For this review, take the finished solid that the model builds, in its own axes (mm). Face numbers are marked on the shaded views. Coordinates: 2 decimals unless noted, no trailing zeros. Write each loop counter-clockwise with the first axis right and the second up, starting at its lowest first coordinate (ties: lowest second). Pieces come first, ordered by that corner, then holes. Notation, with made-up numbers: M 5,-4 L 14,-4 A34 cw 14,34 Z; hole C 38.25,67.25 d2. An arc over 180 degrees is marked long. Return JSON: item names as keys, results as strings.
```python
from build123d import *

# Parameters (mm, degrees)
SKETCH_W        = 134
SKETCH_H        = 62
PAD_DEPTH       = 5
SKETCH001_W     = 134
SKETCH001_H     = 3
PAD001_DEPTH    = 57
SKETCH002_W     = 7
SKETCH002_H     = 17
PAD002_DEPTH    = 7
POCKET_DEPTH    = 89
FILLET_R        = 3
SKETCH004_W     = 3
SKETCH004_H     = 57
PAD003_DEPTH    = 5
SKETCH005_W     = 3
SKETCH005_H     = 7
PAD004_DEPTH    = 3
SKETCH006_R     = 1.75
POCKET001_DEPTH = 134.001
SKETCH007_R     = 1.75
POCKET002_DEPTH = 5
SKETCH008_R     = 1.75
POCKET003_DEPTH = 5
SKETCH009_W     = 3
SKETCH009_H     = 6
PAD005_DEPTH    = 6
SKETCH010_R     = 1.75
POCKET004_DEPTH = 134.001
FILLET001_R     = 3
FILLET002_R     = 2
FILLET003_R     = 3
FILLET004_R     = 2
FILLET005_R     = 6
FILLET006_R     = 6
FILLET007_R     = 2
FILLET008_R     = 0.5
FILLET009_R     = 2
FILLET010_R     = 0.5
FILLET011_R     = 2
FILLET012_R     = 0.5
FILLET013_R     = 2
FILLET014_R     = 0.5
SKETCH011_R     = 1.75
POCKET005_DEPTH = 5
SKETCH012_R     = 2.1
POCKET006_DEPTH = 5
POCKET007_DEPTH = 5
FILLET015_R     = 1
FILLET016_R     = 1


with BuildPart() as part:
    # Sketch → Pad (new body)
    with BuildSketch(Plane.XY):
        with Locations((67, -31)):
            Rectangle(SKETCH_W, SKETCH_H)
    extrude(amount=PAD_DEPTH)

    # Sketch001 (on Face6 of Pad) → Pad001 (join)
    with BuildSketch(Plane.XY.offset(5)):
        with Locations((67, -1.5)):
            Rectangle(SKETCH001_W, SKETCH001_H)
    extrude(amount=PAD001_DEPTH)

    # Sketch002 (on Face11 of Pad001) → Pad002 (join)
    with BuildSketch(Plane.XZ.offset(3)):
        with Locations((26, 53.5)):
            Rectangle(SKETCH002_W, SKETCH002_H)
        with Locations((108, 53.5)):
            Rectangle(SKETCH002_W, SKETCH002_H)
    extrude(amount=PAD002_DEPTH)

    # Sketch003 (on Face14 of Pad002) → Pocket (cut)
    with BuildSketch(Plane(origin=(22.5, 0, 0), x_dir=(0, -1, 0), z_dir=(-1, 0, 0))):
        Polygon((3, 45), (10, 57), (10, 45), align=None)
    extrude(amount=-POCKET_DEPTH, mode=Mode.SUBTRACT)

    # Fillet
    fillet_edges = [part.edges().sort_by_distance(p)[0] for p in [
        (104.5, -10, 59.5),
        (111.5, -10, 59.5),
        (111.5, -6.5, 51),
        (104.5, -6.5, 51),
        (22.5, -10, 59.5),
        (29.5, -10, 59.5),
        (29.5, -6.5, 51),
        (22.5, -6.5, 51),
    ]]
    fillet(fillet_edges, radius=FILLET_R)

    # Sketch004 (on Face1 of Fillet) → Pad003 (join)
    with BuildSketch(Plane.XZ.offset(3)):
        with Locations((1.5, 33.5)):
            Rectangle(SKETCH004_W, SKETCH004_H)
        with Locations((132.5, 33.5)):
            Rectangle(SKETCH004_W, SKETCH004_H)
    extrude(amount=PAD003_DEPTH)

    # Sketch005 (on Face32 of Pad003) → Pad004 (join)
    with BuildSketch(Plane.XZ.offset(8)):
        with Locations((1.5, 8.5)):
            Rectangle(SKETCH005_W, SKETCH005_H)
        with Locations((1.5, 58.5)):
            Rectangle(SKETCH005_W, SKETCH005_H)
        with Locations((132.5, 8.5)):
            Rectangle(SKETCH005_W, SKETCH005_H)
        with Locations((132.5, 58.5)):
            Rectangle(SKETCH005_W, SKETCH005_H)
    extrude(amount=PAD004_DEPTH)

    # Sketch006 (on Face44 of Pad004) → Pocket001 (cut, through all)
    with BuildSketch(Plane(origin=(0, 0, 0), x_dir=(0, -1, 0), z_dir=(-1, 0, 0))):
        with Locations((7, 8)):
            Circle(SKETCH006_R)
    extrude(amount=-POCKET001_DEPTH, mode=Mode.SUBTRACT)

    # Sketch007 (on Face46 of Pocket001) → Pocket002 (cut)
    with BuildSketch(Plane(origin=(0, 0, 0), x_dir=(0, -1, 0), z_dir=(-1, 0, 0))):
        with Locations((7, 58)):
            Circle(SKETCH007_R)
    extrude(amount=-POCKET002_DEPTH, mode=Mode.SUBTRACT)

    # Sketch008 (on Face45 of Pocket002) → Pocket003 (cut)
    with BuildSketch(Plane.YZ.offset(134)):
        with Locations((-7, 58)):
            Circle(SKETCH008_R)
    extrude(amount=-POCKET003_DEPTH, mode=Mode.SUBTRACT)

    # Sketch009 (on Face10 of Pocket003) → Pad005 (join)
    with BuildSketch(Plane.XY.offset(5)):
        with Locations((1.5, -59)):
            Rectangle(SKETCH009_W, SKETCH009_H)
        with Locations((132.5, -59)):
            Rectangle(SKETCH009_W, SKETCH009_H)
    extrude(amount=PAD005_DEPTH)

    # Sketch010 (on Face60 of Pad005) → Pocket004 (cut, through all)
    with BuildSketch(Plane.YZ.offset(134)):
        with Locations((-59, 8)):
            Circle(SKETCH010_R)
    extrude(amount=-POCKET004_DEPTH, mode=Mode.SUBTRACT)

    # Fillet001
    fillet001_edges = [part.edges().sort_by_distance(p)[0] for p in [
        (132.5, -56, 11),
    ]]
    fillet(fillet001_edges, radius=FILLET001_R)

    # Fillet002
    fillet002_edges = [part.edges().sort_by_distance(p)[0] for p in [
        (132.5, -56, 5),
    ]]
    fillet(fillet002_edges, radius=FILLET002_R)

    # Fillet003
    fillet003_edges = [part.edges().sort_by_distance(p)[0] for p in [
        (1.5, -56, 11),
    ]]
    fillet(fillet003_edges, radius=FILLET003_R)

    # Fillet004
    fillet004_edges = [part.edges().sort_by_distance(p)[0] for p in [
        (1.5, -56, 5),
    ]]
    fillet(fillet004_edges, radius=FILLET004_R)

    # Fillet005
    fillet005_edges = [part.edges().sort_by_distance(p)[0] for p in [
        (1.5, -11, 5),
    ]]
    fillet(fillet005_edges, radius=FILLET005_R)

    # Fillet006
    fillet006_edges = [part.edges().sort_by_distance(p)[0] for p in [
        (132.5, -11, 5),
    ]]
    fillet(fillet006_edges, radius=FILLET006_R)

    # Fillet007
    fillet007_edges = [part.edges().sort_by_distance(p)[0] for p in [
        (1.5, -8, 12),
    ]]
    fillet(fillet007_edges, radius=FILLET007_R)

    # Fillet008
    fillet008_edges = [part.edges().sort_by_distance(p)[0] for p in [
        (1.5, -11, 12),
    ]]
    fillet(fillet008_edges, radius=FILLET008_R)

    # Fillet009
    fillet009_edges = [part.edges().sort_by_distance(p)[0] for p in [
        (132.5, -8, 12),
    ]]
    fillet(fillet009_edges, radius=FILLET009_R)

    # Fillet010
    fillet010_edges = [part.edges().sort_by_distance(p)[0] for p in [
        (132.5, -11, 12),
    ]]
    fillet(fillet010_edges, radius=FILLET010_R)

    # Fillet011
    fillet011_edges = [part.edges().sort_by_distance(p)[0] for p in [
        (1.5, -8, 55),
    ]]
    fillet(fillet011_edges, radius=FILLET011_R)

    # Fillet012
    fillet012_edges = [part.edges().sort_by_distance(p)[0] for p in [
        (1.5, -11, 55),
    ]]
    fillet(fillet012_edges, radius=FILLET012_R)

    # Fillet013
    fillet013_edges = [part.edges().sort_by_distance(p)[0] for p in [
        (132.5, -8, 55),
    ]]
    fillet(fillet013_edges, radius=FILLET013_R)

    # Fillet014
    fillet014_edges = [part.edges().sort_by_distance(p)[0] for p in [
        (132.5, -11, 55),
    ]]
    fillet(fillet014_edges, radius=FILLET014_R)

    # Sketch011 (on Face13 of Fillet014) → Pocket005 (cut)
    with BuildSketch(Plane.XY.offset(5)):
        with Locations((19, -8.5)):
            Circle(SKETCH011_R)
        with Locations((19, -53.5)):
            Circle(SKETCH011_R)
        with Locations((119, -53.5)):
            Circle(SKETCH011_R)
        with Locations((119, -8.5)):
            Circle(SKETCH011_R)
    extrude(amount=-POCKET005_DEPTH, mode=Mode.SUBTRACT)

    # Sketch012 (on Face73 of Pocket005) → Pocket006 (cut)
    with BuildSketch(Plane.XY.offset(62)):
        with Locations((26, -6.5)):
            Circle(SKETCH012_R)
        with Locations((108, -6.5)):
            Circle(SKETCH012_R)
    extrude(amount=-POCKET006_DEPTH, mode=Mode.SUBTRACT)

    # Sketch013 (on Face47 of Pocket006) → Pocket007 (cut)
    with BuildSketch(Plane(origin=(0, 0, 0), x_dir=(1, 0, 0), z_dir=(0, 0, -1))):
        with BuildLine():
            ThreePointArc((25, 47), (22.87868, 46.12132), (22, 44))
            Line((22, 20), (22, 44))
            ThreePointArc((22, 20), (22.87868, 17.87868), (25, 17))
            Line((34, 17), (25, 17))
            ThreePointArc((34, 17), (36.12132, 17.87868), (37, 20))
            Line((37, 44), (37, 20))
            ThreePointArc((37, 44), (36.12132, 46.12132), (34, 47))
            Line((25, 47), (34, 47))
        make_face()
    extrude(amount=-POCKET007_DEPTH, mode=Mode.SUBTRACT)

    # Fillet015
    fillet015_edges = [part.edges().sort_by_distance(p)[0] for p in [
        (22, -32, 0),
        (22.87868, -46.12132, 0),
        (29.5, -47, 0),
        (36.12132, -46.12132, 0),
        (37, -32, 0),
        (36.12132, -17.87868, 0),
        (29.5, -17, 0),
        (22.87868, -17.87868, 0),
    ]]
    fillet(fillet015_edges, radius=FILLET015_R)

    # Fillet016
    fillet016_edges = [part.edges().sort_by_distance(p)[0] for p in [
        (22, -32, 5),
        (22.87868, -17.87868, 5),
        (29.5, -17, 5),
        (36.12132, -17.87868, 5),
        (37, -32, 5),
        (36.12132, -46.12132, 5),
        (29.5, -47, 5),
        (22.87868, -46.12132, 5),
    ]]
    fillet(fillet016_edges, radius=FILLET016_R)


solid = part.part
```
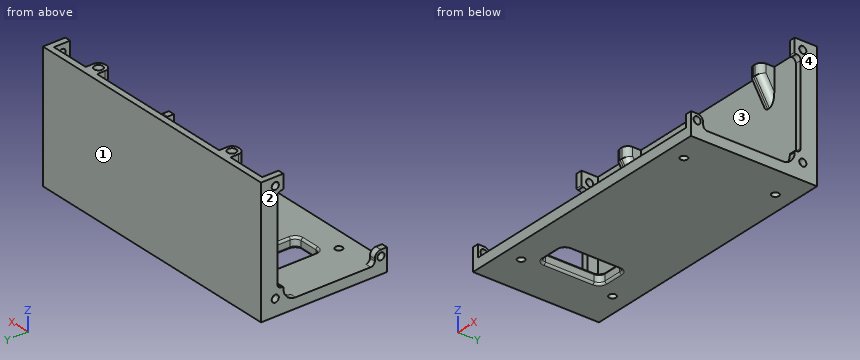
1. We need section C-C (x = 101). State the section outline as (y, z) points, plus the area to 3 significant figures.
Checks:
{"outline": "M -62,0 L 0,0 L 0,62 L -3,62 L -3,5 L -62,5 Z", "area": "481 mm2"}
2. Wall thickness on L1, parallel to Y at x = 119, z = 3.2; L2, parallel to Z at x = 132.4, y = -7; L3, parallel to Y at x = 26, z = 58: over which ranges is each line inside the solid? List them lowest first. Write a range as from..to.
Checks:
{"L1": "-62..-55.25, -51.75..-10.25, -6.75..0", "L2": "0..6.25, 9.75..56.25, 59.75..62", "L3": "-10..-8.6, -4.4..0"}
3. Draft analysis for pull direction X (two halves, no side actions). For the marked faces 1, 2, 3 and 4, state which applies: +X half, -X half, draft (parallel to the pull), parting line (faces both ways), or undercut.
Checks:
{"face 1": "draft", "face 2": "-X half", "face 3": "undercut", "face 4": "+X half"}
4. We need section B-B (z = 17.5). State the section outline as (x, y) points.
Checks:
{"outline": "M 0,-8 L 3,-8 L 3,-3 L 131,-3 L 131,-8 L 134,-8 L 134,0 L 0,0 Z"}
5. We need section A-A (x = 119). State the section outline as (y, z) points.
Checks:
{"outline": "M -62,0 L -55.25,0 L -55.25,5 L -62,5 Z; M -51.75,0 L -10.25,0 L -10.25,5 L -51.75,5 Z; M -6.75,0 L 0,0 L 0,62 L -3,62 L -3,5 L -6.75,5 Z"}
6. Clearance check with flat-ended pins moving along their axes: pin 1 Ø3 at (y, z) = (-7, 8) entering from +X; pin 2 Ø3.5 at (x, z) = (1.5, 59) entering from -Y; pin 3 Ø1.5 at (x, y) = (133, -60.5) entering from +Z; pin 4 Ø5.5 at (x, y) = (19, -53.5) entering from +Z. State where each tip first meets the part, or that it passes through.
Checks:
{"pin 1": "through", "pin 2": "y = -11", "pin 3": "z = 11", "pin 4": "z = 5"}
